from build123d import *

# Parameters (mm, degrees)
SKETCH2_R           = 201
BOSS_EXTRUDE1_DEPTH = 750
SHELL1_T            = -10
SKETCH3_R           = 192.25
CUT_EXTRUDE1_DEPTH  = 793.718108788
FILLET2_R           = 2
FILLET3_R           = 2


with BuildPart() as part:
    # Sketch2 → Boss-Extrude1 (new body)
    with BuildSketch(Plane.XY):
        Circle(SKETCH2_R)
    extrude(amount=BOSS_EXTRUDE1_DEPTH)

    # Shell1
    shell1_openings = [part.faces().sort_by_distance(p)[0] for p in [
        (0, 0, 750),
    ]]
    offset(amount=SHELL1_T, openings=shell1_openings, kind=Kind.INTERSECTION)

    # Sketch3 → Cut-Extrude1 (cut, through all)
    with BuildSketch(Plane.XY.offset(10)):
        Circle(SKETCH3_R)
    extrude(amount=-CUT_EXTRUDE1_DEPTH, mode=Mode.SUBTRACT)

    # Fillet2
    fillet2_edges = [part.edges().sort_by_distance(p)[0] for p in [
        (-201, 0, 0),
    ]]
    fillet(fillet2_edges, radius=FILLET2_R)

    # Fillet3
    fillet3_edges = [part.edges().sort_by_distance(p)[0] for p in [
        (-201, 0, 750),
    ]]
    fillet(fillet3_edges, radius=FILLET3_R)


solid = part.part
Could you check a few things on this model? Use its own coordinates, in mm. Give positions to 0.01 mm unless a question says otherwise; leave off trailing zeros. Order: outer loops, then holes, each group sorted by start corner. A loop starts at its lowest first (then second) coordinate and runs counter-clockwise, first axis right, second up.
1. Suppose I cut it at C-C (z = 61). List the corners of the cut face in (x, y) for me, plus the area to 3 significant figures.
2. Will these pins go through, and if not, where does the flat tip stop? P1, Ø12, axis at x = -131.5, z = 420, coming from the +Y side; P2, Ø5, axis at y = 47, z = 255.5, coming from the +X side; P3, Ø1, axis at x = -14.5, z = 484, coming from the -Y side.
3. Suppose I cut it at A-A (y = 0). List the corners of the cut face in (x, z) for me.
4. We'd pull the mould along X, two halves only. Please class faces 1 (the flat face through (-163, 104, 0)), 2 (the cylindrical face through (108.06, 169.48, 369.78)), 3 (the cylindrical face through (183.37, 57.75, 5.07)), 4 (the cylindrical face through (-41.405, -186.458, 374.82)): pulls with the +X half, pulls with the -X half, needs draft (parallel to the pull), parting line crosses it, or undercut.
5. I need wall thicknesses on L1, parallel to Y at x = 0, z = 7; L2, parallel to Y at x = 0, z = 435; L3, parallel to Z at x = -181, y = -61.5. Which ranges of each line are inside material? Lowest first, please.
Solved:
1. outline: circle Ø402 at (0, 0); hole circle Ø382 at (0, 0)
1. area: 12,300 mm2
2. P1: stops at y = 157.01
2. P2: stops at x = 196.01
2. P3: stops at y = -200.51
3. outline: (-201, 2) arc R2 ccw to (-199, 0) - (-192.25, 0) - (-192.25, 10) - (-191, 10) - (-191, 750) - (-199, 750) arc R2 ccw to (-201, 748) - close; (191, 10) - (192.25, 10) - (192.25, 0) - (199, 0) arc R2 ccw to (201, 2) - (201, 748) arc R2 ccw to (199, 750) - (191, 750) - close
4. face 1: needs draft
4. face 2: parting line crosses it
4. face 3: undercut
4. face 4: undercut
5. L1: y = -201 to -192.25, 192.25 to 201
5. L2: y = -201 to -191, 191 to 201
5. L3: z = 10 to 750
